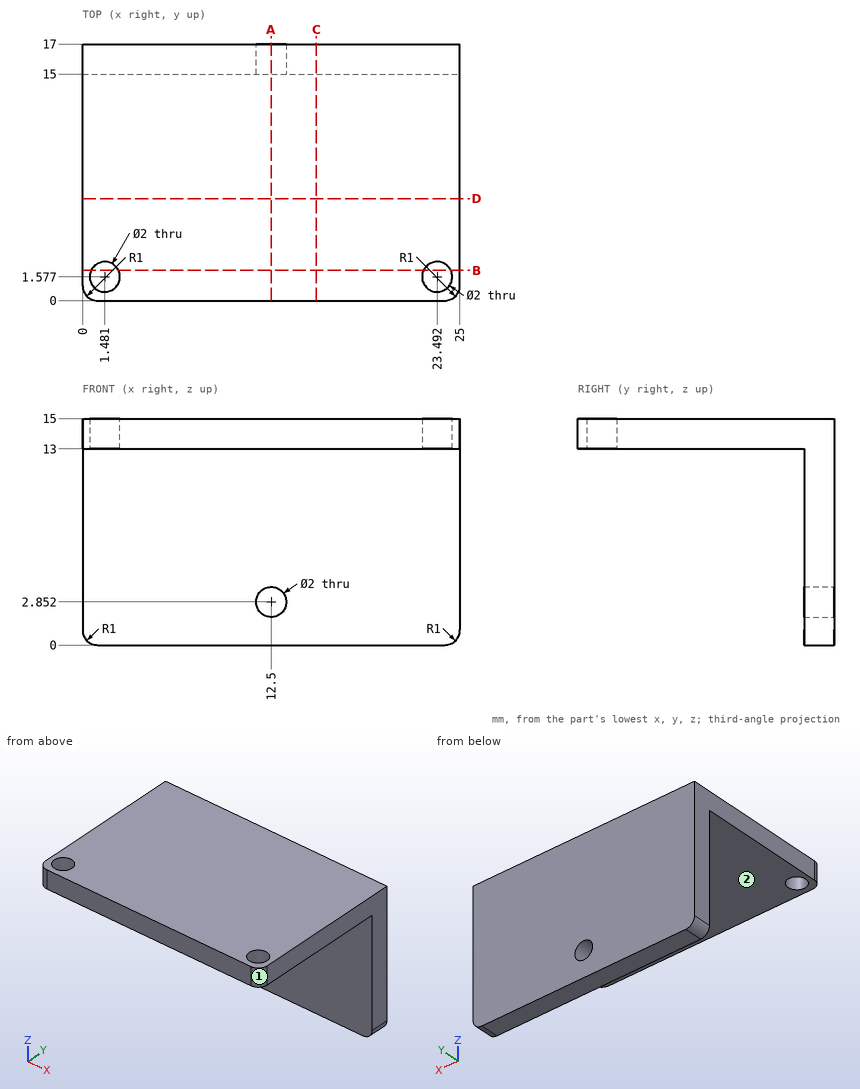
Study the drawing (mm; zero at the part's minimum x, y, z) and answer. A direction names the side the tool comes from. Round coordinates to 2 decimals unless told otherwise and drop trailing zeros. Loops run counter-clockwise (first coordinate to the right, second up) from the corner with the lowest first, then second, coordinate; pieces in that order, holes last. Notation, with made-up numbers: (57, 29) - (97, 29) arc R22 cw to (97, 67) - close; hole circle Ø8 at (63, 63). An arc over 180 degrees is marked (long way). Use one line per item in the form item = value. Start each with the question number.
1. The part is cut by section A-A on x = 12.5. Determine the outline of the cut face in (y, z), then the cut area to 3 significant figures.
2. Consider line 1 (Z direction, x = 12.5, y = 15.6); line 2 (Y direction, x = 15.5, z = 12.75); line 3 (Z direction, x = 10, y = 14.75). Determine where each line is inside the solid, lowest interval first. Write a range as [from, to].
3. The part is cut by section D-D on y = 6.75. Determine the outline of the cut face in (x, z), then the cut area to 3 significant figures.
4. A tool of negligible diameter and unlimited length cuts with its end or side. For the marked faces 1 and 2, from which of +Z, -Z, +X, -X, +Y, -Y can it reach the whole face along a straight path? Write none if from no direction.
5. The part is cut by section C-C on x = 15.5. Determine the outline of the cut face in (y, z), then the cut area to 3 significant figures.
6. The part is cut by section B-B on y = 2. Determine the outline of the cut face in (x, z) (1 decimal).
7. Given pin 1 Ø1.5 at (x, z) = (9.5, 9.5) entering from -Y; pin 2 Ø7.5 at (x, y) = (11.5, 11) entering from -Z, each flat-ended and moving along its own axis, determine where each tip first touches the part or whether it passes through.
Geometry check:
q1.outline = (0, 13) - (15, 13) - (15, 3.85) - (17, 3.85) - (17, 15) - (0, 15) - close; (15, 0) - (17, 0) - (17, 1.85) - (15, 1.85) - close
q1.area = 56.0 mm^2
q2.line_1 = [0, 1.85], [3.85, 15]
q2.line_2 = [15, 17]
q2.line_3 = [13, 15]
q3.outline = (0, 13) - (25, 13) - (25, 15) - (0, 15) - close
q3.area = 50.0 mm^2
q4.face_1 = +Z, -Z, +X, -Y
q4.face_2 = -Z, +X, -X, -Y
q5.outline = (0, 13) - (15, 13) - (15, 0) - (17, 0) - (17, 15) - (0, 15) - close
q5.area = 60.0 mm^2
q6.outline = (0, 13) - (0.6, 13) - (0.6, 15) - (0, 15) - close; (2.4, 13) - (22.6, 13) - (22.6, 15) - (2.4, 15) - close; (24.4, 13) - (25, 13) - (25, 15) - (24.4, 15) - close
q7.pin_1 = 15
q7.pin_2 = 13
